The model under review builds one solid part; all positions refer to its coordinate system, in mm. Round coordinates to 2 decimals unless told otherwise and drop trailing zeros. Loops run counter-clockwise (first coordinate to the right, second up) from the corner with the lowest first, then second, coordinate; pieces in that order, holes last. Notation, with made-up numbers: M -38,65 L -11,65 A14 cw -11,70 Z; hole C 9.5,-23 d2. An arc over 180 degrees is marked long. Answer as a JSON object with one key per item and string values. Group by question number.
Item 1: Consider section D-D (z = 128.5). Give the boundary of the cut face in (x, y), and give its area (3 significant figures).
Item 2: Consider section B-B (z = 225). Give the boundary of the cut face in (x, y).
Item 3: Consider section C-C (y = 4). Give the boundary of the cut face in (x, z), and give its area (3 significant figures).
Item 4: Insertion check: P1, Ø1, axis at x = 2, z = 198.5, coming from the +Y side. The pin has a flat end and moves straight along its axis. Give the tip position at first contact, or say it passes through.
Item 5: To check wall thickness, follow line 1 (X direction, y = 1.5, z = 161); line 2 (X direction, y = 7.25, z = 169); line 3 (Y direction, x = 0.5, z = 132). State the ranges of each line that lie inside material, in increasing order.
Item 6: Consider section A-A (x = 0). Give the boundary of the cut face in (y, z).
```python
from build123d import *

# Parameters (mm, degrees)
EXTRUDE_1_DEPTH          = 245
SKETCH_2_R               = 2.5
CUT_EXTRUDE_1_DEPTH      = 246.21623111
CUT_EXTRUDE_2_DEPTH      = 246.21623111
CUT_EXTRUDE_2_DEPTH_BACK = 246.21623111
SKETCH_3_W               = 10
SKETCH_3_H               = 100


with BuildPart() as part:
    # ｽｹｯﾁ1 → ﾎﾞｽ - 押し出し1 (new body)
    with BuildSketch(Plane.XY):
        Polygon((-5, 9), (-5, 0), (5, 0), (5, 9), (3, 9), (3, 2), (-3, 2), (-3, 9), align=None)
    extrude(amount=EXTRUDE_1_DEPTH)

    # ｽｹｯﾁ2 → ｶｯﾄ - 押し出し1 (cut, through all)
    with BuildSketch(Plane.XZ):
        with Locations(Location((0, 225, 0), (0, 0, 270))):
            Circle(SKETCH_2_R)
        with Locations(Location((0, 217, 0), (0, 0, 270))):
            Circle(SKETCH_2_R)
        with Locations(Location((0, 122.5, 0), (0, 0, 270))):
            Circle(SKETCH_2_R)
        with Locations(Location((0, 209, 0), (0, 0, 270))):
            Circle(SKETCH_2_R)
        with Locations(Location((0, 193, 0), (0, 0, 270))):
            Circle(SKETCH_2_R)
        with Locations(Location((0, 161, 0), (0, 0, 270))):
            Circle(SKETCH_2_R)
    cut_extrude_1 = extrude(amount=-CUT_EXTRUDE_1_DEPTH, mode=Mode.SUBTRACT)

    # ﾐﾗｰ1: ｶｯﾄ - 押し出し1 across plane
    add(cut_extrude_1.mirror(Plane.XY.offset(122.5)), mode=Mode.SUBTRACT)

    # ｽｹｯﾁ3 → ｶｯﾄ - 押し出し2 (cut, two sides: drawn at the far end of the back side and taken through both)
    with BuildSketch(Plane.XZ.offset(-CUT_EXTRUDE_2_DEPTH_BACK)):
        with Locations((0, 50)):
            Rectangle(SKETCH_3_W, SKETCH_3_H)
    extrude(amount=CUT_EXTRUDE_2_DEPTH + CUT_EXTRUDE_2_DEPTH_BACK, mode=Mode.SUBTRACT)


solid = part.part
```
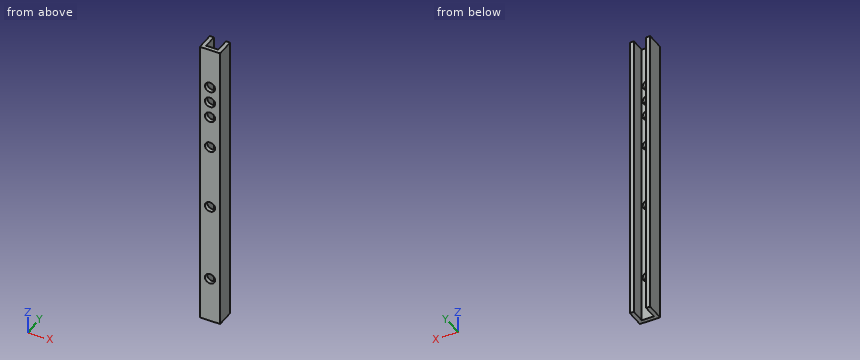
Geometry results:
{
 "1": {"outline": "M -5,0 L 5,0 L 5,9 L 3,9 L 3,2 L -3,2 L -3,9 L -5,9 Z", "area": "48.0 mm^2"},
 "2": {"outline": "M -5,0 L -2.5,0 L -2.5,2 L -3,2 L -3,9 L -5,9 Z; M 2.5,0 L 5,0 L 5,9 L 3,9 L 3,2 L 2.5,2 Z"},
 "3": {"outline": "M -5,100 L -3,100 L -3,245 L -5,245 Z; M 3,100 L 5,100 L 5,245 L 3,245 Z", "area": "580 mm^2"},
 "4": {"P1": "stops at y = 2"},
 "5": {"line 1": "x = -5 to -2.5, 2.5 to 5", "line 2": "x = -5 to -3, 3 to 5", "line 3": "y = 0 to 2"},
 "6": {"outline": "M 0,100 L 2,100 L 2,120 L 0,120 Z; M 0,125 L 2,125 L 2,158.5 L 0,158.5 Z; M 0,163.5 L 2,163.5 L 2,190.5 L 0,190.5 Z; M 0,195.5 L 2,195.5 L 2,206.5 L 0,206.5 Z; M 0,211.5 L 2,211.5 L 2,214.5 L 0,214.5 Z; M 0,219.5 L 2,219.5 L 2,222.5 L 0,222.5 Z; M 0,227.5 L 2,227.5 L 2,245 L 0,245 Z"}
}
